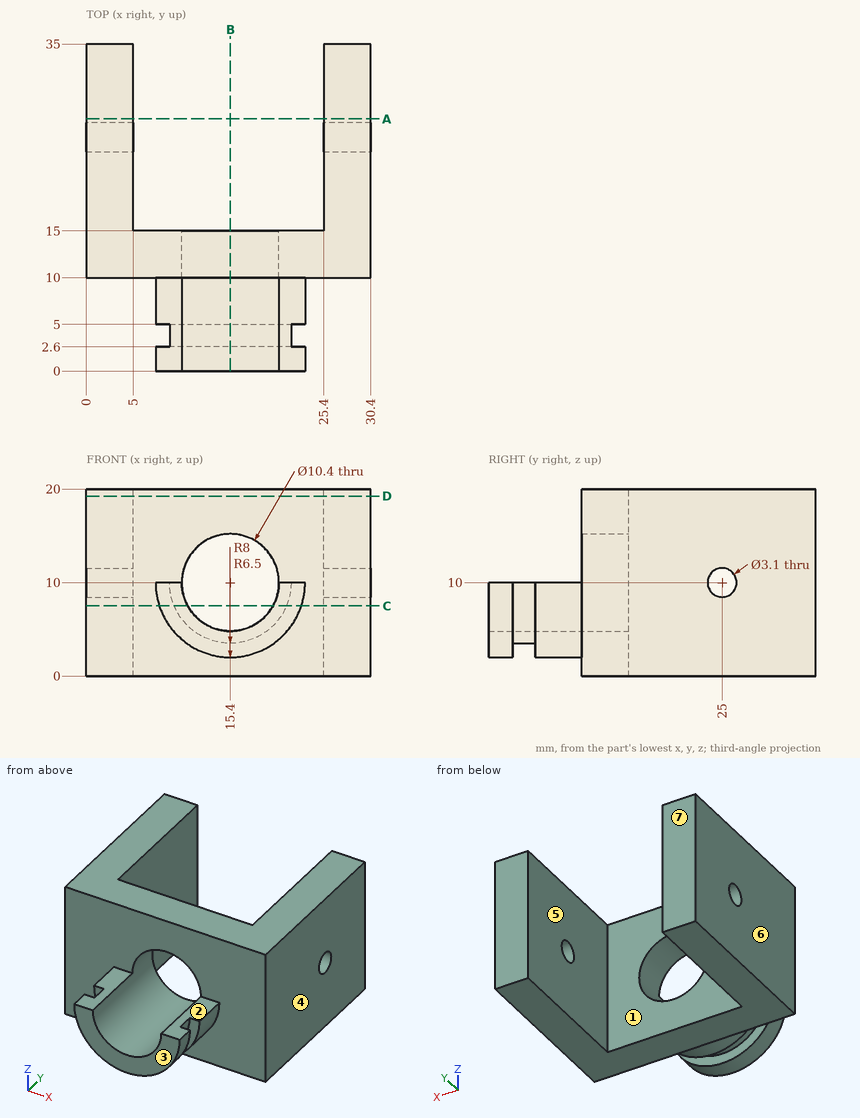
Print and shaded views of the part. All mm, measured from the part's lowest x, y and z. A direction names the side the tool comes from. Give positions to 0.01 mm unless a question says otherwise; leave off trailing zeros. Loops run counter-clockwise (first coordinate to the right, second up) from the corner with the lowest first, then second, coordinate; pieces in that order, holes last.
1) Wall check: line 1 (Z direction, x = 27, y = 25); line 2 (X direction, y = 30.5, z = 7); line 3 (Y direction, x = 8, z = 18). Give the ranges that are in metal, low to high.
2) Saw through at C-C (z = 7.5). Write the cut outline in (x, y).
3) Tool access for the marked faces 1, 2 and 3: list every direction of +Z, -Z, +X, -X, +Y, -Y with a clear straight run to the whole face (end or side of a thin tool).
4) Pull direction X, two halves, no side cores. Call the marked faces 4, 5, 6 and 7: +X half, -X half, draft (parallel to the pull), parting line (faces both ways), or undercut.
5) Saw through at D-D (z = 19.25). Write the cut outline in (x, y), plus the area to 3 significant figures.
6) Saw through at B-B (x = 15.4). Write the cut outline in (y, z).
7) Saw through at A-A (y = 27). Write the cut outline in (x, z), plus the area to 3 significant figures.
8) Flat gauge pins, fed straight in: pin 1 Ø4 at (x, z) = (15.5, 6) entering from +Y; pin 2 Ø1.9 at (y, z) = (25, 10) entering from +X; pin 3 Ø6 at (x, z) = (4.5, 17.5) entering from -Y; pin 4 Ø0.8 at (x, y) = (8.5, 6) entering from +Z. Where does each tip first touch, or does it go through?
Answer block:
1. line 1: z = 0 to 8.45, 11.55 to 20
1. line 2: x = 0 to 5, 25.4 to 30.4
1. line 3: y = 10 to 15
2. outline: (0, 10) - (7.8, 10) - (7.8, 5) - (9.4, 5) - (9.4, 2.6) - (7.8, 2.6) - (7.8, 0) - (10.84, 0) - (10.84, 15) - (5, 15) - (5, 35) - (0, 35) - close; (19.96, 0) - (23, 0) - (23, 2.6) - (21.4, 2.6) - (21.4, 5) - (23, 5) - (23, 10) - (30.4, 10) - (30.4, 35) - (25.4, 35) - (25.4, 15) - (19.96, 15) - close
3. face 1: +Z, -Z, +Y
3. face 2: +Z, +X, -X, -Y
3. face 3: +Z, -Z, +X, -X, -Y
4. face 4: +X half
4. face 5: undercut
4. face 6: -X half
4. face 7: draft
5. outline: (0, 10) - (30.4, 10) - (30.4, 35) - (25.4, 35) - (25.4, 15) - (5, 15) - (5, 35) - (0, 35) - close
5. area: 352 mm2
6. outline: (0, 2) - (2.6, 2) - (2.6, 3.5) - (5, 3.5) - (5, 2) - (10, 2) - (10, 0) - (15, 0) - (15, 4.8) - (0, 4.8) - close; (10, 15.2) - (15, 15.2) - (15, 20) - (10, 20) - close
7. outline: (0, 0) - (5, 0) - (5, 20) - (0, 20) - close; (25.4, 0) - (30.4, 0) - (30.4, 20) - (25.4, 20) - close
7. area: 200 mm2
8. pin 1: stops at y = 15
8. pin 2: passes through
8. pin 3: stops at y = 10
8. pin 4: stops at z = 10
